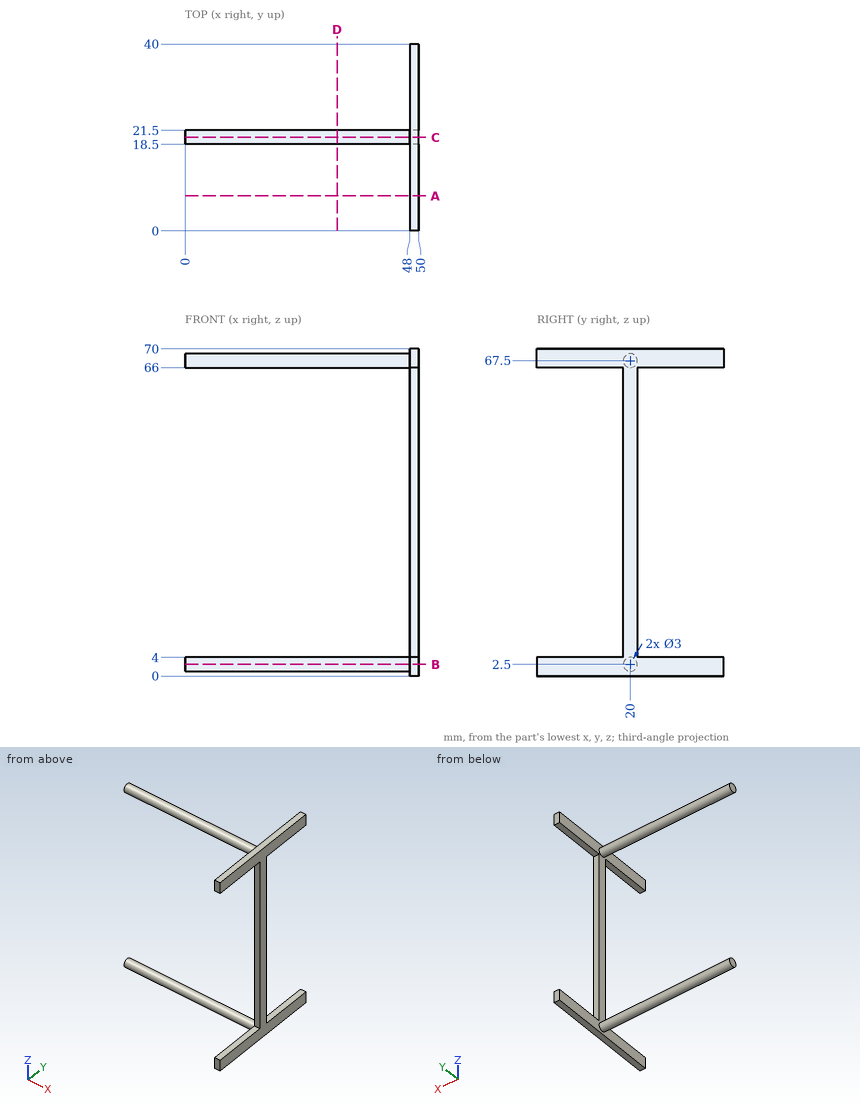
The figure shows three views and two pictorial views of one solid part (mm, origin at its lowest corner). Answer the questions. Give positions to 0.01 mm unless a question says otherwise; leave off trailing zeros. Order: outer loops, then holes, each group sorted by start corner. A loop starts at its lowest first (then second) coordinate and runs counter-clockwise, first axis right, second up. Notation, with made-up numbers: (-16, 87) -> (9, 87) arc R30 cw to (9, 112) -> close; hole circle Ø4 at (77, 83). An arc over 180 degrees is marked (long way). Answer as a JSON object with one key per item and string values. Group by question number.
Item 1: The part is cut by section C-C on y = 20. Write down the section's boundary in (x, z), and give its area (3 significant figures).
Item 2: The part is cut by section D-D on x = 32.5. Write down the section's boundary in (y, z), and give its area (3 significant figures).
Item 3: Consider L1, parallel to Z at x = 12.5, y = 20; L2, parallel to Z at x = 43, y = 20.5; L3, parallel to X at y = 20, z = 17. Determine where each line is inside the solid, lowest interval first. Write a range as from..to.
Item 4: The part is cut by section A-A on y = 7.5. Write down the section's boundary in (x, z).
Item 5: Flat-ended cylindrical pins translate along their axes: pin 1 (20 mm diameter, centred on y = 22.5, z = 46.5, fed in from -X); pin 2 (1 mm diameter, centred on x = 49, z = 50.5, fed in from +Y); pin 3 (1 mm diameter, centred on x = 49, y = 32, fed in from -Z); pin 4 (12 mm diameter, centred on x = 27, y = 20, fed in from +Z). Find the tip coordinate at first contact, or state that the pin passes through.
Item 6: The part is cut by section B-B on z = 2.5. Write down the section's boundary in (x, y).
Result set:
{
 "1": {"outline": "(0, 1) -> (48, 1) -> (48, 0) -> (50, 0) -> (50, 70) -> (48, 70) -> (48, 69) -> (0, 69) -> (0, 66) -> (48, 66) -> (48, 4) -> (0, 4) -> close", "area": "428 mm²"},
 "2": {"outline": "circle Ø3 at (20, 2.5); circle Ø3 at (20, 67.5)", "area": "14.1 mm²"},
 "3": {"L1": "1..4, 66..69", "L2": "1.09..3.91, 66.09..68.91", "L3": "48..50"},
 "4": {"outline": "(48, 0) -> (50, 0) -> (50, 4) -> (48, 4) -> close; (48, 66) -> (50, 66) -> (50, 70) -> (48, 70) -> close"},
 "5": {"pin 1": "x = 48", "pin 2": "y = 21.5", "pin 3": "z = 0", "pin 4": "z = 69"},
 "6": {"outline": "(0, 18.5) -> (48, 18.5) -> (48, 0) -> (50, 0) -> (50, 40) -> (48, 40) -> (48, 21.5) -> (0, 21.5) -> close"}
}
